Could you check a few things on this model? Use its own coordinates, in mm. Give positions to 0.01 mm unless a question says otherwise; leave off trailing zeros. Order: outer loops, then holes, each group sorted by start corner. A loop starts at its lowest first (then second) coordinate and runs counter-clockwise, first axis right, second up.
from build123d import *

# Parameters (mm, degrees)
F0_W     = 226.934572
F0_H     = 226.934572
F0_R     = 1.7272
F0_W_2   = 19.558
F0_H_2   = 40.64
F0_R_2   = 1.25
F1_DEPTH = 5.08


with BuildPart() as f1:
    # F0 (on Top) → F1 (new body)
    with BuildSketch(Plane.XY):
        Rectangle(F0_W, F0_H)
        with Locations((-107.117286, -104.450286)):
            Circle(F0_R, mode=Mode.SUBTRACT)
        with Locations((-89.337286, -104.450286)):
            Circle(F0_R, mode=Mode.SUBTRACT)
        with Locations((-107.117286, -80.574286)):
            Circle(F0_R, mode=Mode.SUBTRACT)
        with Locations((-89.337286, -80.574286)):
            Circle(F0_R, mode=Mode.SUBTRACT)
        Rectangle(F0_W_2, F0_H_2, mode=Mode.SUBTRACT)
        with Locations((89.337286, -104.450286)):
            Circle(F0_R, mode=Mode.SUBTRACT)
        with Locations((107.117286, -104.450286)):
            Circle(F0_R, mode=Mode.SUBTRACT)
        with Locations((89.337286, -80.574286)):
            Circle(F0_R, mode=Mode.SUBTRACT)
        with Locations((107.117286, -80.574286)):
            Circle(F0_R, mode=Mode.SUBTRACT)
        with Locations((106.167276, -4.750003)):
            Circle(F0_R_2, mode=Mode.SUBTRACT)
        with Locations((-107.117286, 80.574286)):
            Circle(F0_R, mode=Mode.SUBTRACT)
        with Locations((-89.337286, 80.574286)):
            Circle(F0_R, mode=Mode.SUBTRACT)
        with Locations((-107.117286, 104.450286)):
            Circle(F0_R, mode=Mode.SUBTRACT)
        with Locations((-89.337286, 104.450286)):
            Circle(F0_R, mode=Mode.SUBTRACT)
        with Locations((106.167276, 4.750003)):
            Circle(F0_R_2, mode=Mode.SUBTRACT)
        with Locations((89.337286, 80.574286)):
            Circle(F0_R, mode=Mode.SUBTRACT)
        with Locations((107.117286, 80.574286)):
            Circle(F0_R, mode=Mode.SUBTRACT)
        with Locations((89.337286, 104.450286)):
            Circle(F0_R, mode=Mode.SUBTRACT)
        with Locations((107.117286, 104.450286)):
            Circle(F0_R, mode=Mode.SUBTRACT)
    extrude(amount=F1_DEPTH)


solid = f1.part
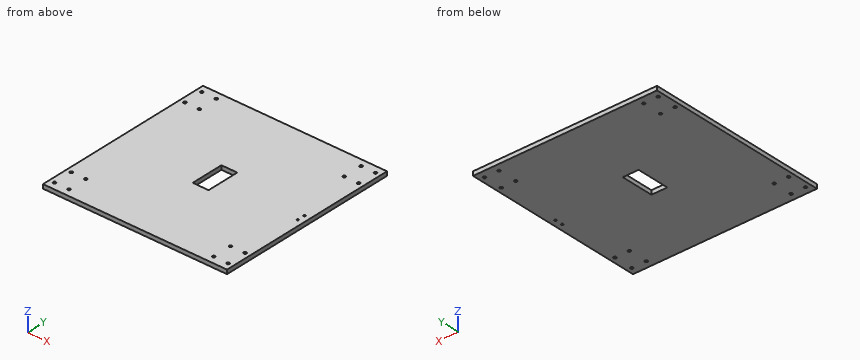
Item 1: Imagine slicing it at B-B on z = 3.45. Give the number of separate pieces and of enclosed holes in the cut face, then the cut area to 3 significant figures.
Findings:
separate pieces: 1
enclosed holes: 19
area: 50,500 mm2
Item 2: Please list where these lines run through material, in increasing order: line 1 along X through (y, z) = (5, 1.1); line 2 along X through (y, z) = (18.5, 4.5); line 3 along Y through (x, z) = (9.5, 2.9).
Findings:
line 1: x = -113.47 to -9.78, 9.78 to 104.94, 107.39 to 113.47
line 2: x = -113.47 to -9.78, 9.78 to 113.47
line 3: y = -113.47 to -20.32, 20.32 to 113.47
Item 3: Imagine slicing it at A-A on y = -13. List the corners of the cut face in (x, z) for me.
Findings:
outline: (-113.47, 0) - (-9.78, 0) - (-9.78, 5.08) - (-113.47, 5.08) - close; (9.78, 0) - (113.47, 0) - (113.47, 5.08) - (9.78, 5.08) - close
Item 4: For pin 1 (5.5 mm diameter, centred on x = 89.34, y = -104.45, fed in from +Z), with a flat end and sliding along its axis, tell me the tip position at first contact or that it passes through.
Findings:
pin 1: stops at z = 5.08
